Here's how the part is built. I have some questions about the finished solid (model axes, mm). Face numbers are marked on the shaded views. A direction names the side the tool comes from. Round coordinates to 2 decimals unless told otherwise and drop trailing zeros. Loops run counter-clockwise (first coordinate to the right, second up) from the corner with the lowest first, then second, coordinate; pieces in that order, holes last. Notation, with made-up numbers: M -31.75,77.25 L 19.25,77.25 A23 cw 19.25,95.25 Z; hole C 12,77 d6. An arc over 180 degrees is marked long. Answer as a JSON object with one key per item and string values.
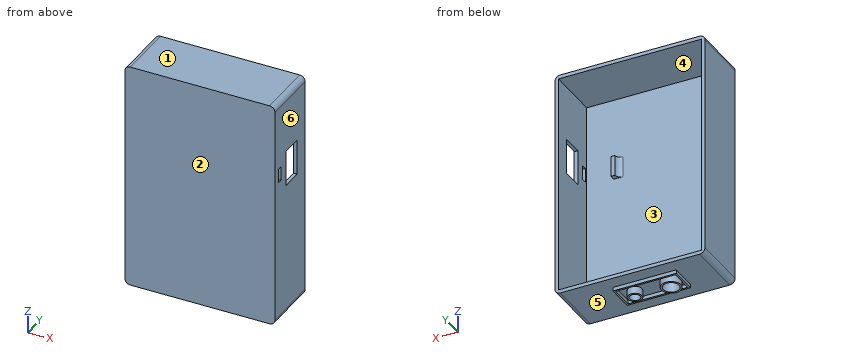
from build123d import *

# Parameters (mm, degrees)
SKETCH1_W           = 83
SKETCH1_H           = 126.35
BOSS_EXTRUDE1_DEPTH = 2
SKETCH2_W           = 83
SKETCH2_H           = 126.35
SKETCH2_W_2         = 79
SKETCH2_H_2         = 122.35
BOSS_EXTRUDE2_DEPTH = 30
SKETCH3_W           = 7.8
SKETCH3_H           = 2.9
SKETCH3_W_2         = 19.74
SKETCH3_H_2         = 12.02
CUT_EXTRUDE1_DEPTH  = 108.59219593
SKETCH4_W           = 2.167162511
SKETCH4_H           = 11.452793886
BOSS_EXTRUDE3_DEPTH = 3
FILLET2_R           = 3
FILLET1_R           = 3
SKETCH6_R           = 4.4
SKETCH6_R_2         = 2.85
CUT_EXTRUDE2_DEPTH  = 135.941366897
SKETCH7_W           = 35
SKETCH7_H           = 15
SKETCH7_W_2         = 33
SKETCH7_H_2         = 13
SKETCH7_R           = 5.4
SKETCH7_R_2         = 4.4
SKETCH7_R_3         = 3.85
SKETCH7_R_4         = 2.85
BOSS_EXTRUDE4_DEPTH = 2
SKETCH8_R           = 3.85
SKETCH8_R_2         = 2.85
SKETCH8_R_3         = 5.4
SKETCH8_R_4         = 4.4
BOSS_EXTRUDE5_DEPTH = 2


with BuildPart() as part:
    # Sketch1 → Boss-Extrude1 (new body)
    with BuildSketch(Plane(origin=(0, 0, 0), x_dir=(1, 0, 0), z_dir=(0, 1, 0))):
        Rectangle(SKETCH1_W, SKETCH1_H)
    extrude(amount=BOSS_EXTRUDE1_DEPTH)

    # Sketch2 → Boss-Extrude2 (add)
    with BuildSketch(Plane(origin=(0, 2, 0), x_dir=(1, 0, 0), z_dir=(0, 1, 0))):
        Rectangle(SKETCH2_W, SKETCH2_H)
        Rectangle(SKETCH2_W_2, SKETCH2_H_2, mode=Mode.SUBTRACT)
    extrude(amount=BOSS_EXTRUDE2_DEPTH)

    # Sketch3 → Cut-Extrude1 (cut, through all)
    with BuildSketch(Plane.ZY.offset(-39.5)):
        with Locations((21.175, 4.99)):
            Rectangle(SKETCH3_W, SKETCH3_H)
        with Locations((21.175, 17.45)):
            Rectangle(SKETCH3_W_2, SKETCH3_H_2)
    extrude(amount=-CUT_EXTRUDE1_DEPTH, mode=Mode.SUBTRACT)

    # Sketch4 → Boss-Extrude3 (add)
    with BuildSketch(Plane(origin=(0, 2, 0), x_dir=(1, 0, 0), z_dir=(0, 1, 0))):
        with Locations((23.516418745, -21.175)):
            Rectangle(SKETCH4_W, SKETCH4_H)
    extrude(amount=BOSS_EXTRUDE3_DEPTH)

    # Fillet2
    fillet2_edges = [part.edges().sort_by_distance(p)[0] for p in [
        (22.432837489, 2, 21.175),
    ]]
    fillet(fillet2_edges, radius=FILLET2_R - 0.0001)  # a hair under: the kernel refuses the full size

    # Fillet1
    fillet1_edges = [part.edges().sort_by_distance(p)[0] for p in [
        (-41.5, 16, -63.175),
        (-41.5, 16, 63.175),
        (41.5, 16, 63.175),
        (41.5, 16, -63.175),
    ]]
    fillet(fillet1_edges, radius=FILLET1_R)

    # Sketch6 → Cut-Extrude2 (cut, through all)
    with BuildSketch(Plane.XY.offset(-61.175)):
        with Locations((-15, 17)):
            Circle(SKETCH6_R)
        with Locations((5, 17)):
            Circle(SKETCH6_R_2)
    extrude(amount=-CUT_EXTRUDE2_DEPTH, mode=Mode.SUBTRACT)

    # Sketch7 → Boss-Extrude4 (add)
    # profile 1 of 3: a face of its own
    with BuildSketch(Plane(origin=(0, 0, -63.175), x_dir=(-1, 0, 0), z_dir=(0, 0, -1))):
        with Locations((4.225, 17)):
            Rectangle(SKETCH7_W, SKETCH7_H)
        with Locations((4.225, 17)):
            Rectangle(SKETCH7_W_2, SKETCH7_H_2, mode=Mode.SUBTRACT)
    # profile 2 of 3: a face of its own
    with BuildSketch(Plane(origin=(0, 0, -63.175), x_dir=(-1, 0, 0), z_dir=(0, 0, -1))):
        with Locations((15, 17)):
            Circle(SKETCH7_R)
        with Locations(Location((15, 17, 0), (0, 0, 180))):
            Circle(SKETCH7_R_2, mode=Mode.SUBTRACT)
    # profile 3 of 3: a face of its own
    with BuildSketch(Plane(origin=(0, 0, -63.175), x_dir=(-1, 0, 0), z_dir=(0, 0, -1))):
        with Locations((-5, 17)):
            Circle(SKETCH7_R_3)
        with Locations(Location((-5, 17, 0), (0, 0, 180))):
            Circle(SKETCH7_R_4, mode=Mode.SUBTRACT)
    extrude(amount=BOSS_EXTRUDE4_DEPTH)

    # Sketch8 → Boss-Extrude5 (add)
    # profile 1 of 2: a face of its own
    with BuildSketch(Plane(origin=(0, 0, -65.175), x_dir=(-1, 0, 0), z_dir=(0, 0, -1))):
        with Locations((-5, 17)):
            Circle(SKETCH8_R)
        with Locations(Location((-5, 17, 0), (0, 0, 180))):
            Circle(SKETCH8_R_2, mode=Mode.SUBTRACT)
    # profile 2 of 2: a face of its own
    with BuildSketch(Plane(origin=(0, 0, -65.175), x_dir=(-1, 0, 0), z_dir=(0, 0, -1))):
        with Locations((15, 17)):
            Circle(SKETCH8_R_3)
        with Locations(Location((15, 17, 0), (0, 0, 180))):
            Circle(SKETCH8_R_4, mode=Mode.SUBTRACT)
    extrude(amount=BOSS_EXTRUDE5_DEPTH)


solid = part.part
Item 1: We'd pull the mould along Z, two halves only. Please class the marked faces 1, 2 and 3: +Z half, -Z half, draft (parallel to the pull), parting line (faces both ways), or undercut.
Solution:
{"face 1": "+Z half", "face 2": "draft", "face 3": "undercut"}
Item 2: If I drill on L1, parallel to Y at x = -15, z = -63.6; L2, parallel to X at y = 6.5, z = -48.5; L3, parallel to Y at x = 5, z = -65.4, over which ranges is the centre line in solid material (lowest first)? Write a range as from..to.
Solution:
{"L1": "y = 9.5..10.5, 11.6..12.6, 21.4..22.4, 23.5..24.5", "L2": "x = -41.5..-39.5, 39.5..41.5", "L3": "y = 13.15..14.15, 19.85..20.85"}
Item 3: I want a section at C-C on x = -5.5. List the corners of the cut face in (y, z) for me (3 decimals).
Solution:
{"outline": "M 0,-63.175 L 9.5,-63.175 L 9.5,-65.175 L 10.5,-65.175 L 10.5,-63.175 L 23.5,-63.175 L 23.5,-65.175 L 24.5,-65.175 L 24.5,-63.175 L 32,-63.175 L 32,-61.175 L 2,-61.175 L 2,61.175 L 32,61.175 L 32,63.175 L 0,63.175 Z"}
Item 4: For P1, Ø1.6, axis at x = 40.5, y = 5.5, coming from the -Z side; P2, Ø3, axis at x = 2.5, z = 0.5, coming from the +Y side; P3, Ø2.5, axis at x = 21, y = 3.5, coming from the -Z side (3 decimals), each with a flat end and sliding along its axis, tell me the tip position at first contact or that it passes through.
Solution:
{"P1": "stops at z = -62.92", "P2": "stops at y = 2", "P3": "stops at z = -63.175"}
Item 5: I want a section at B-B on x = -15. List the corners of the cut face in (y, z) for me (3 decimals), plus the area to 3 significant figures.
Solution:
{"outline": "M 0,-63.175 L 9.5,-63.175 L 9.5,-65.175 L 10.5,-65.175 L 10.5,-63.175 L 11.6,-63.175 L 11.6,-67.175 L 12.6,-67.175 L 12.6,-61.175 L 2,-61.175 L 2,61.175 L 32,61.175 L 32,63.175 L 0,63.175 Z; M 21.4,-67.175 L 22.4,-67.175 L 22.4,-63.175 L 23.5,-63.175 L 23.5,-65.175 L 24.5,-65.175 L 24.5,-63.175 L 32,-63.175 L 32,-61.175 L 21.4,-61.175 Z", "area": "367 mm2"}
Item 6: I want a section at D-D on z = -39. List the corners of the cut face in (x, y) for me, plus the area to 3 significant figures.
Solution:
{"outline": "M -41.5,0 L 41.5,0 L 41.5,32 L 39.5,32 L 39.5,2 L -39.5,2 L -39.5,32 L -41.5,32 Z", "area": "286 mm2"}
Item 7: I want a section at A-A on z = 22. Count the separate pieces of the cut face and the enclosed holes in it, plus the area to 3 significant figures.
Solution:
{"separate pieces": "3", "enclosed holes": "0", "area": "265 mm2"}
Item 8: For the marked faces 4, 5 and 6, which set-ups out of +Z, -Z, +X, -X, +Y, -Y let a thin tool reach every point of the face, with its end or its side?
Solution:
{"face 4": "+Y", "face 5": "-Z", "face 6": "+Z, -Z, +X, +Y, -Y"}
